from build123d import *

# Parameters (mm, degrees)
SKETCH2_W           = 30
SKETCH2_H           = 27
BOSS_EXTRUDE1_DEPTH = 20
SKETCH6_W           = 6
SKETCH6_H           = 26
CUT_EXTRUDE4_DEPTH  = 26
SKETCH9_W           = 5
SKETCH9_H           = 15
CUT_EXTRUDE5_DEPTH  = 21
SKETCH11_R          = 5
CUT_EXTRUDE8_DEPTH  = 0.5
SKETCH12_W          = 2.75
SKETCH12_H          = 11
CUT_EXTRUDE12_DEPTH = 17.5
SKETCH15_R          = 4.5
CUT_EXTRUDE13_DEPTH = 6


with BuildPart() as part:
    # Sketch2 → Boss-Extrude1 (new body)
    with BuildSketch(Plane(origin=(0, 0, 0), x_dir=(0, 0, -1), z_dir=(1, 0, 0))):
        with Locations((15, 13.5)):
            Rectangle(SKETCH2_W, SKETCH2_H)
    extrude(amount=BOSS_EXTRUDE1_DEPTH)

    # Sketch6 → Cut-Extrude4 (cut)
    with BuildSketch(Plane(origin=(2.296116437, 27, -0.293484995), x_dir=(1, 0, 0), z_dir=(0, 1, 0))):
        with Locations((12.365844825, 15.206515005)):
            Rectangle(SKETCH6_W, SKETCH6_H)
    extrude(amount=-CUT_EXTRUDE4_DEPTH, mode=Mode.SUBTRACT)

    # Sketch9 → Cut-Extrude5 (cut)
    with BuildSketch(Plane(origin=(0, 27, 0), x_dir=(1, 0, 0), z_dir=(0, 1, 0))):
        with Locations((9.161961261, 14)):
            Rectangle(SKETCH9_W, SKETCH9_H)
    extrude(amount=-CUT_EXTRUDE5_DEPTH, mode=Mode.SUBTRACT)

    # Sketch11 → Cut-Extrude8 (cut)
    with BuildSketch(Plane.ZY):
        with Locations((-15.1, 13.5)):
            Circle(SKETCH11_R)
    extrude(amount=-CUT_EXTRUDE8_DEPTH, mode=Mode.SUBTRACT)

    # Sketch12 → Cut-Extrude12 (cut)
    with BuildSketch(Plane(origin=(0, 27, 0), x_dir=(1, 0, 0), z_dir=(0, 1, 0))):
        with Locations((4.286961261, 15.5)):
            Rectangle(SKETCH12_W, SKETCH12_H)
    extrude(amount=-CUT_EXTRUDE12_DEPTH, mode=Mode.SUBTRACT)

    # Sketch15 → Cut-Extrude13 (cut)
    with BuildSketch(Plane.ZY.offset(-0.5)):
        with Locations((-15.04, 13.5)):
            Circle(SKETCH15_R)
    extrude(amount=-CUT_EXTRUDE13_DEPTH, mode=Mode.SUBTRACT)


solid = part.part
Check sheet for the modelled part. Datum: model origin and axes. Units: mm. A direction names the side the tool comes from. Give positions to 0.01 mm unless a question says otherwise; leave off trailing zeros. Loops run counter-clockwise (first coordinate to the right, second up) from the corner with the lowest first, then second, coordinate; pieces in that order, holes last. Notation, with made-up numbers: M 17.25,-27.75 L 36.25,-27.75 A23 cw 36.25,-9.75 Z; hole C 3,24.5 d1. An arc over 180 degrees is marked long. Return JSON: item names as keys, results as strings. Group by question number.
1. Cross-section at D-D on y = 24.75. Record the boundary of the cut face in (x, z), plus the area to 3 significant figures.
2. Tool access check on faces 4 (the flat face through (4, 9.5, -19)), 5 (the flat face through (10, 0, -15)), 6 (the flat face through (6.5, 14, -15)). Record the directions out of +Z, -Z, +X, -X, +Y, -Y that give a thin tool (end or side, any length) a straight path to the whole face; none if there is none.
3. Go/stop test with flat-tipped pins: pin 1 (1.5 mm diameter, centred on x = 12.5, z = -15, fed in from +Y); pin 2 (5 mm diameter, centred on x = 16, y = 12, fed in from +Z); pin 3 (3 mm diameter, centred on x = 10.5, z = -11.5, fed in from +Y); pin 4 (5 mm diameter, centred on y = 13, z = -16, fed in from -X). Record where each tip stops, or that it passes through.
4. Cross-section at A-A on y = 4. Record the boundary of the cut face in (x, z), plus the area to 3 significant figures.
5. Thickness scan on L1, parallel to X at y = 19.25, z = -6.25; L2, parallel to X at y = 12.5, z = -18.25; L3, parallel to X at y = 20, z = -17. Record the ranges inside material, lowest first.
6. Cross-section at C-C on x = 5. Record the boundary of the cut face in (y, z).
7. Cross-section at B-B on z = -18. Record the boundary of the cut face in (x, y), plus the area to 3 significant figures.
8. Mould release check, pull along X, two halves, no side actions. Record for faces 1 (the flat face through (10, 13, 0)), 2 (the flat face through (20, 14, -15)), 3 (the flat face through (5.662, 20, -15)): released by +X, released by -X, zero draft, split by the parting line, or undercut.
Return value:
{
 "1": {"outline": "M 0,-30 L 20,-30 L 20,0 L 0,0 Z; hole M 2.91,-21 L 5.66,-21 L 5.66,-10 L 2.91,-10 Z; hole M 6.66,-21.5 L 11.66,-21.5 L 11.66,-28.5 L 17.66,-28.5 L 17.66,-2.5 L 11.66,-2.5 L 11.66,-6.5 L 6.66,-6.5 Z", "area": "339 mm^2"},
 "2": {"face 4": "+Y", "face 5": "+Z, -Z, +X, -X, -Y", "face 6": "-X"},
 "3": {"pin 1": "y = 1", "pin 2": "z = 0", "pin 3": "y = 6", "pin 4": "x = 6.5"},
 "4": {"outline": "M 0,-30 L 20,-30 L 20,0 L 0,0 Z; hole M 11.66,-28.5 L 17.66,-28.5 L 17.66,-2.5 L 11.66,-2.5 Z", "area": "444 mm^2"},
 "5": {"L1": "0 to 11.66, 17.66 to 20", "L2": "6.5 to 6.66, 17.66 to 20", "L3": "0 to 2.91, 5.66 to 6.66, 17.66 to 20"},
 "6": {"outline": "M 0,-30 L 27,-30 L 27,-21 L 9.5,-21 L 9.5,-17.1 A4.5 cw 9.5,-12.98 L 9.5,-10 L 27,-10 L 27,0 L 0,0 Z"},
 "7": {"outline": "M 0,0 L 20,0 L 20,27 L 17.66,27 L 17.66,1 L 11.66,1 L 11.66,6 L 6.66,6 L 6.66,27 L 5.66,27 L 5.66,16.89 L 6.5,16.89 L 6.5,10.11 L 5.66,10.11 L 5.66,9.5 L 2.91,9.5 L 2.91,10.11 L 0.5,10.11 L 0.5,9.43 L 0,9.43 Z; M 0,17.57 L 0.5,17.57 L 0.5,16.89 L 2.91,16.89 L 2.91,27 L 0,27 Z", "area": "205 mm^2"},
 "8": {"face 1": "zero draft", "face 2": "released by +X", "face 3": "undercut"}
}
